Model file for the job. Use its own axes, mm. A direction names the side the tool comes from. Coordinates: 2 decimals unless noted, no trailing zeros. Loops run counter-clockwise (first coordinate to the right, second up) from the corner with the lowest first, then second, coordinate; pieces in that order, holes last.
from build123d import *

# Parameters (mm, degrees)
F3_DEPTH  = 1
F4_R      = 3.25
F5_DEPTH  = 2.001
F8_DEPTH  = 2
F10_DEPTH = 27.001


with BuildPart() as f1:
    # F0 (on Front) → F1 (revolve)
    with BuildSketch(Plane.XZ):
        with BuildLine():
            Line((0, 32), (0, 35))
            Line((0, 35), (-8, 35))
            Line((-8, 35), (-8, 32))
            ThreePointArc((-8, 32), (-12.379208, 16.766787), (-24.179687, 6.184872))
            ThreePointArc((-24.179687, 6.184872), (-26.236652, 4.340318), (-27, 1.684987))
            Line((-27, 1.684987), (-27, 0))
            Line((-27, 0), (-25, 0))
            Line((-25, 0), (-25, 1.684987))
            ThreePointArc((-25, 1.684987), (-24.541991, 3.278186), (-23.307813, 4.384918))
            ThreePointArc((-23.307813, 4.384918), (-10.684547, 15.704655), (-6, 32))
            Line((-6, 32), (0, 32))
        make_face()
    revolve(axis=Axis((0, 0, 17.5), (0, 0, -1)))

    # F2 (on face) → F3 (cut)
    with BuildSketch(Plane(origin=(0, 0, 32), x_dir=(1, 0, 0), z_dir=(0, 0, -1))):
        Polygon((4.25, -2.453739), (4.25, 2.453739), (0, 4.907477), (-4.25, 2.453739), (-4.25, -2.453739), (0, -4.907477), align=None)
    extrude(amount=-F3_DEPTH, mode=Mode.SUBTRACT)

    # F4 (on face) → F5 (cut, through all)
    with BuildSketch(Plane(origin=(0, 0, 33), x_dir=(1, 0, 0), z_dir=(0, 0, -1))):
        Circle(F4_R)
    extrude(amount=-F5_DEPTH, mode=Mode.SUBTRACT)

    # F7 (on offset) → F8 (join)
    with BuildSketch(Plane(origin=(0, 0, 1), x_dir=(1, 0, 0), z_dir=(0, 0, -1))):
        with BuildLine():
            Line((5.5, -9.526279), (12.5, -21.650635))
            ThreePointArc((12.5, -21.650635), (25, 0), (12.5, 21.650635))
            Line((12.5, 21.650635), (5.5, 9.526279))
            ThreePointArc((5.5, 9.526279), (11, 0), (5.5, -9.526279))
        make_face()
        with BuildLine():
            ThreePointArc((-12.5, 21.650635), (-25, 0), (-12.5, -21.650635))
            Line((-12.5, -21.650635), (-5.5, -9.526279))
            ThreePointArc((-5.5, -9.526279), (-11, 0), (-5.5, 9.526279))
            Line((-5.5, 9.526279), (-12.5, 21.650635))
        make_face()
    extrude(amount=-F8_DEPTH)

    # F9 (on Front) → F10 (cut, through all)
    with BuildSketch(Plane.XZ):
        with BuildLine():
            Line((1.75, 0), (1.75, 2))
            ThreePointArc((1.75, 2), (0, 3.75), (-1.75, 2))
            Line((-1.75, 2), (-1.75, 0))
            Line((-1.75, 0), (1.75, 0))
        make_face()
    extrude(amount=-F10_DEPTH, mode=Mode.SUBTRACT)


solid = f1.part
Q1. Slice it at B-B (z = 27). List the corners of the cut face in (x, y), and give its area (3 significant figures).
Answers:
outline: circle Ø16.88 at (0, 0); hole circle Ø12.82 at (0, 0)
area: 94.7 mm2
Q2. Which spindle directions (+Z, -Z, +X, -X, +Y, -Y) get a long thin tool onto all of the face, cutting with end or side? Do faces 4 (the flat face through (2.095, 3.698, 32.493)), 5 (the flat face through (15, 0, 3)), 6 (the flat face through (8, -24, 0)), 7 (the flat face through (1.75, 26, 1)), 8 (the cylindrical face through (-2.579, 1.978, 33.986)). Say none if no direction does.
Answers:
face 4: -Z
face 5: none
face 6: -Z, +X, -X, +Y, -Y
face 7: -Z, +Y
face 8: +Z, -Z
Q3. Slice it at A-A (z = 9). List the corners of the cut face in (x, y).
Answers:
outline: circle Ø39.09 at (0, 0); hole circle Ø32.75 at (0, 0)
Q4. Mould opens along X. For faces 1 (the cylindrical face through (1.73, -7.81, 33.48)), 2 (the flat face through (2, 3, 33)), 3 (the flat face through (3.4, 0.1, 35)) say: +X half, -X half, draft (parallel to the pull), parting line (faces both ways), or undercut.
Answers:
face 1: parting line
face 2: undercut
face 3: draft
Q5. Drill centre lines: line 1 (Y direction, x = 0, z = 33.9); line 2 (X direction, y = 0, z = 0.6); line 3 (Y direction, x = -9, z = 4.5). Where is each one in solid material? Low to high.
Answers:
line 1: y = -8 to -3.25, 3.25 to 8
line 2: x = -27 to -25, 25 to 27
line 3: y = -24.53 to -21.25, 21.25 to 24.53
Q6. Flat gauge pins, fed straight in: P1, Ø5, axis at y = 2, z = 18, coming from the -X side; P2, Ø6, axis at x = 17.5, y = 1, coming from the +Z side; P3, Ø10, axis at x = -16.5, y = 14.5, coming from the +Z side. Where does each tip first touch, or does it go through?
Answers:
P1: stops at x = -13.1
P2: stops at z = 13.78
P3: stops at z = 11.17
